Part print with two shaded views. Sizes in mm from the minimum x, y, z corner. A direction names the side the tool comes from. Give positions to 0.01 mm unless a question says otherwise; leave off trailing zeros. Loops run counter-clockwise (first coordinate to the right, second up) from the corner with the lowest first, then second, coordinate; pieces in that order, holes last. Notation, with made-up numbers: M 68,-21 L 122,-21 A16 cw 122,-9 Z; hole C 38,25 d11. An arc over 180 degrees is marked long. Answer in a Markdown table with one row per item.
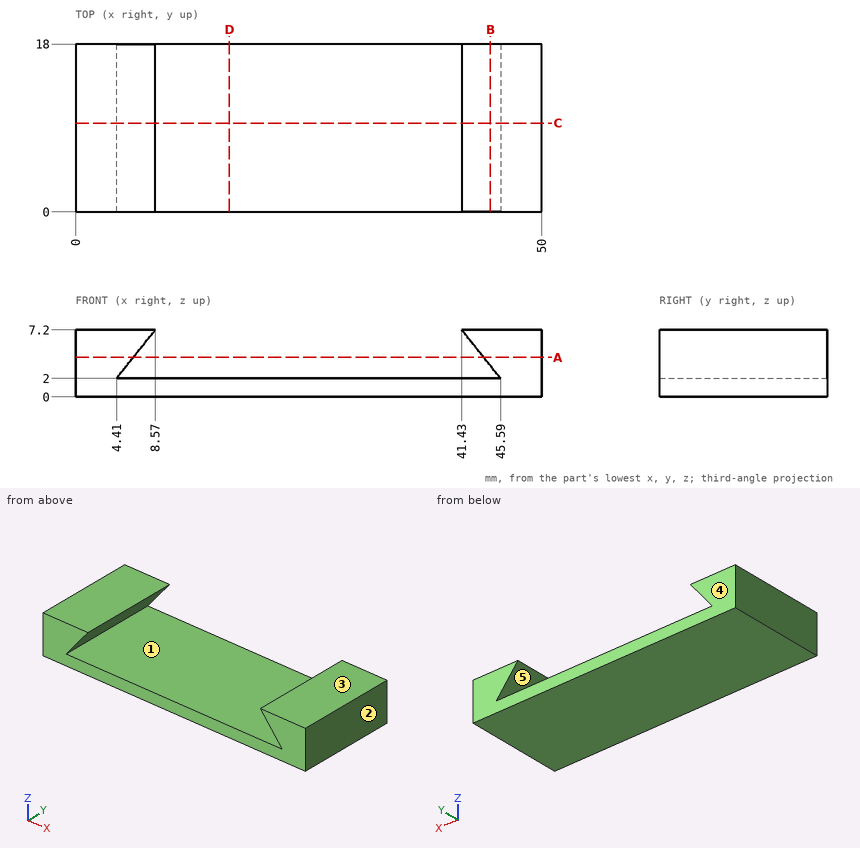
Q1. Mould opens along X. For the marked faces 1, 2 and 3 say: released by +X, released by -X, zero draft, split by the parting line, or undercut.
Reported:
| item | result |
|---|---|
| face 1 | undercut |
| face 2 | released by +X |
| face 3 | zero draft |
Q2. Drop flat-ended pins along their axis: pin 1 (10 mm diameter, centred on x = 39.5, y = 11, fed in from +Z); pin 2 (5.5 mm diameter, centred on x = 17.5, y = 5.5, fed in from +Z). Give the stop position or say it passes through.
Reported:
| item | result |
|---|---|
| pin 1 | z = 7.2 |
| pin 2 | z = 2 |
Q3. Saw through at D-D (x = 16.5). Give the cut face in (y, z), and give its area (3 significant figures).
Reported:
| item | result |
|---|---|
| outline | M 0,0 L 18,0 L 18,2 L 0,2 Z |
| area | 36.0 mm² |
Q4. Saw through at A-A (z = 4.25). Give the cut face in (x, y).
Reported:
| item | result |
|---|---|
| outline | M 0,0 L 6.21,0 L 6.21,18 L 0,18 Z; M 43.79,0 L 50,0 L 50,18 L 43.79,18 Z |
Q5. Saw through at C-C (y = 9.5). Give the cut face in (x, z).
Reported:
| item | result |
|---|---|
| outline | M 0,0 L 50,0 L 50,7.2 L 41.43,7.2 L 45.59,2 L 4.41,2 L 8.57,7.2 L 0,7.2 Z |
Q6. Saw through at B-B (x = 44.5). Give the cut face in (y, z), and give its area (3 significant figures).
Reported:
| item | result |
|---|---|
| outline | M 0,0 L 18,0 L 18,2 L 0,2 Z; M 0,3.36 L 18,3.36 L 18,7.2 L 0,7.2 Z |
| area | 105 mm² |
Q7. Probe probe 1 along Z at (x, y) = (33, 10); probe 2 along X at (y, z) = (11.75, 5); probe 3 along X at (y, z) = (15, 4). List the from-to ranges inside material, lowest first.
Reported:
| item | result |
|---|---|
| probe 1 | 0 to 2 |
| probe 2 | 0 to 6.81, 43.19 to 50 |
| probe 3 | 0 to 6.01, 43.99 to 50 |
Q8. 3-axis set-ups, long thin cutter, end or side, ignore diameter. For the marked faces 4 and 5: which of +Z, -Z, +X, -X, +Y, -Y reach the whole face in a straight line?
Reported:
| item | result |
|---|---|
| face 4 | +Z, -Z, +X, -X, +Y |
| face 5 | +Y, -Y |
